from build123d import *

# Parameters (mm, degrees)
SKETCH1_W                                = 1524
SKETCH1_H                                = 152.4
BOSS_EXTRUDE1_DEPTH                      = 152.4
BOSS_EXTRUDE2_DEPTH                      = 152.4
FILLET1_R                                = 25.4
SKETCH9_W                                = 152.4
SKETCH9_H                                = 38.1
BOSS_EXTRUDE3_DEPTH                      = 101.6
SKETCH11_W                               = 152.4
SKETCH11_H                               = 38.1
BOSS_EXTRUDE4_DEPTH                      = 56.515
F_0000_CLEARANCE_HOLE1_D                 = 7.874
F_0000_CLEARANCE_HOLE1_DEPTH             = 12.7
F_0000_CLEARANCE_HOLE1_TIP               = 2.365588257
CBORE_FOR_3_4_HEX_HEAD_BOLT1_D           = 19.84248
CBORE_FOR_3_4_HEX_HEAD_BOLT1_CBORE_D     = 41.275
CBORE_FOR_3_4_HEX_HEAD_BOLT1_CBORE_DEPTH = 13.3096


with BuildPart() as part:
    # Sketch1 → Boss-Extrude1 (new body)
    with BuildSketch(Plane.XY):
        with Locations((762, 76.2)):
            Rectangle(SKETCH1_W, SKETCH1_H)
    extrude(amount=BOSS_EXTRUDE1_DEPTH)

    # Sketch8 → Boss-Extrude2 (add)
    with BuildSketch(Plane(origin=(0, 152.4, 0), x_dir=(1, 0, 0), z_dir=(0, 1, 0))):
        Polygon((0, -152.4), (-254, -355.6), (-286.356492461, -355.6), (-286.356492461, -152.4), (0, 0), align=None)
    boss_extrude2 = extrude(amount=-BOSS_EXTRUDE2_DEPTH)

    # Mirror1: Boss-Extrude2 across plane
    add(boss_extrude2.mirror(Plane(origin=(762, 0, 0), x_dir=(0, 0, 1), z_dir=(1, 0, 0))))

    # Fillet1
    # the kernel refuses this fillet: 25.4 mm, written as the material it takes off along each edge
    with BuildSketch(Plane(origin=(-342.412174328, 0, 182.23304427), x_dir=(0, 1, 0), z_dir=(0.882766643577138, 0, -0.4698117207856294))) as fillet1_piece_1:
        with BuildLine():
            CenterArc((FILLET1_R, FILLET1_R), FILLET1_R, 180, 90)
            Line((0, FILLET1_R), (0, 0))
            Line((0, 0), (FILLET1_R, 0))
        make_face()
    extrude(amount=451.385265964, mode=Mode.SUBTRACT)
    with BuildSketch(Plane(origin=(-286.356492461, 0, 419.1), x_dir=(0, 1, 0), z_dir=(0, 0, -1))) as fillet1_piece_2:
        with BuildLine():
            CenterArc((FILLET1_R, FILLET1_R), FILLET1_R, 180, 90)
            Line((0, FILLET1_R), (0, 0))
            Line((0, 0), (FILLET1_R, 0))
        make_face()
    extrude(amount=330.2, mode=Mode.SUBTRACT)
    with BuildSketch(Plane(origin=(49.5851694, 0, 112.73186448), x_dir=(0, 1, 0), z_dir=(-0.780868809443027, 0, 0.6246950475544286))) as fillet1_piece_3_section:
        with BuildLine():
            CenterArc((FILLET1_R, FILLET1_R), FILLET1_R, 180, 90)
            Line((0, FILLET1_R), (0, 0))
            Line((0, 0), (FILLET1_R, 0))
        make_face()
    fillet1_piece_3 = extrude(amount=452.278711262, mode=Mode.PRIVATE)
    fillet1_piece_3 = split(fillet1_piece_3, bisect_by=Plane(origin=(-158.082016781, 5.808462647, 152.4), z_dir=(0, 0, 1)), keep=Keep.TOP, mode=Mode.PRIVATE)
    add(fillet1_piece_3, mode=Mode.SUBTRACT)
    with BuildSketch(Plane(origin=(-63.5, 0, 152.4), x_dir=(0, 1, 0), z_dir=(1, 0, 0))) as fillet1_piece_4_section:
        with BuildLine():
            CenterArc((FILLET1_R, -FILLET1_R), FILLET1_R, 90, 90)
            Line((0, -FILLET1_R), (0, 0))
            Line((0, 0), (FILLET1_R, 0))
        make_face()
    fillet1_piece_4 = extrude(amount=1651, mode=Mode.PRIVATE)
    fillet1_piece_4 = split(fillet1_piece_4, bisect_by=Plane(origin=(467.415014496, 5.779770976, -221.532011596), z_dir=(0.6246950475544286, 0, 0.780868809443027)), keep=Keep.TOP, mode=Mode.PRIVATE)
    fillet1_piece_4 = split(fillet1_piece_4, bisect_by=Plane(origin=(1056.584985505, 5.779770976, -221.532011596), z_dir=(-0.6246950475544286, 0, 0.780868809443027)), keep=Keep.TOP, mode=Mode.PRIVATE)
    add(fillet1_piece_4, mode=Mode.SUBTRACT)
    with BuildSketch(Plane(origin=(1474.4148306, 0, 112.73186448), x_dir=(0, 1, 0), z_dir=(0.780868809443027, 0, 0.6246950475544286))) as fillet1_piece_5_section:
        with BuildLine():
            CenterArc((FILLET1_R, -FILLET1_R), FILLET1_R, 90, 90)
            Line((0, -FILLET1_R), (0, 0))
            Line((0, 0), (FILLET1_R, 0))
        make_face()
    fillet1_piece_5 = extrude(amount=452.278711262, mode=Mode.PRIVATE)
    fillet1_piece_5 = split(fillet1_piece_5, bisect_by=Plane(origin=(1682.082016781, 5.808462647, 152.4), z_dir=(0, 0, 1)), keep=Keep.TOP, mode=Mode.PRIVATE)
    add(fillet1_piece_5, mode=Mode.SUBTRACT)
    with BuildSketch(Plane(origin=(1810.356492461, 0, 419.1), x_dir=(0, 1, 0), z_dir=(0, 0, -1))) as fillet1_piece_6:
        with BuildLine():
            CenterArc((FILLET1_R, -FILLET1_R), FILLET1_R, 90, 90)
            Line((0, -FILLET1_R), (0, 0))
            Line((0, 0), (FILLET1_R, 0))
        make_face()
    extrude(amount=330.2, mode=Mode.SUBTRACT)
    with BuildSketch(Plane(origin=(1866.412174328, 0, 182.23304427), x_dir=(0, 1, 0), z_dir=(-0.882766643577138, 0, -0.4698117207856294))) as fillet1_piece_7:
        with BuildLine():
            CenterArc((FILLET1_R, -FILLET1_R), FILLET1_R, 90, 90)
            Line((0, -FILLET1_R), (0, 0))
            Line((0, 0), (FILLET1_R, 0))
        make_face()
    extrude(amount=451.385265964, mode=Mode.SUBTRACT)
    with BuildSketch(Plane(origin=(-63.5, 0, 0), x_dir=(0, 1, 0), z_dir=(1, 0, 0))) as fillet1_piece_8:
        with BuildLine():
            CenterArc((FILLET1_R, FILLET1_R), FILLET1_R, 180, 90)
            Line((0, FILLET1_R), (0, 0))
            Line((0, 0), (FILLET1_R, 0))
        make_face()
    extrude(amount=1651, mode=Mode.SUBTRACT)
    with BuildSketch(Plane(origin=(-63.5, 0, 152.4), x_dir=(0, 1, 0), z_dir=(1, 0, 0))) as fillet1_piece_9a_section:
        with BuildLine():
            CenterArc((FILLET1_R, -FILLET1_R), FILLET1_R, 90, 90)
            Line((0, -FILLET1_R), (0, 0))
            Line((0, 0), (FILLET1_R, 0))
        make_face()
    fillet1_piece_9a = extrude(amount=1651, mode=Mode.PRIVATE)
    fillet1_piece_9a = split(fillet1_piece_9a, bisect_by=Plane(origin=(-13.902468194, 5.43719391, 163.521974555), z_dir=(-0.6246950475544286, 0, -0.780868809443027)), keep=Keep.TOP, mode=Mode.PRIVATE)
    with BuildSketch(Plane(origin=(49.5851694, 0, 112.73186448), x_dir=(0, 1, 0), z_dir=(-0.780868809443027, 0, 0.6246950475544286))) as fillet1_piece_9b_section:
        with BuildLine():
            CenterArc((FILLET1_R, FILLET1_R), FILLET1_R, 180, 90)
            Line((0, FILLET1_R), (0, 0))
            Line((0, 0), (FILLET1_R, 0))
        make_face()
    fillet1_piece_9b = extrude(amount=452.278711262, mode=Mode.PRIVATE)
    fillet1_piece_9b = split(fillet1_piece_9b, bisect_by=Plane(origin=(17.80384621, 5.43719391, 152.4), z_dir=(0, 0, -1)), keep=Keep.TOP, mode=Mode.PRIVATE)
    fillet1_piece_9 = fillet1_piece_9a & fillet1_piece_9b
    add(fillet1_piece_9, mode=Mode.SUBTRACT)
    with BuildSketch(Plane(origin=(-63.5, 0, 152.4), x_dir=(0, 1, 0), z_dir=(1, 0, 0))) as fillet1_piece_10a_section:
        with BuildLine():
            CenterArc((FILLET1_R, -FILLET1_R), FILLET1_R, 90, 90)
            Line((0, -FILLET1_R), (0, 0))
            Line((0, 0), (FILLET1_R, 0))
        make_face()
    fillet1_piece_10a = extrude(amount=1651, mode=Mode.PRIVATE)
    fillet1_piece_10a = split(fillet1_piece_10a, bisect_by=Plane(origin=(1537.902468194, 5.43719391, 163.521974555), z_dir=(0.6246950475544286, 0, -0.780868809443027)), keep=Keep.TOP, mode=Mode.PRIVATE)
    with BuildSketch(Plane(origin=(1474.4148306, 0, 112.73186448), x_dir=(0, 1, 0), z_dir=(0.780868809443027, 0, 0.6246950475544286))) as fillet1_piece_10b_section:
        with BuildLine():
            CenterArc((FILLET1_R, -FILLET1_R), FILLET1_R, 90, 90)
            Line((0, -FILLET1_R), (0, 0))
            Line((0, 0), (FILLET1_R, 0))
        make_face()
    fillet1_piece_10b = extrude(amount=452.278711262, mode=Mode.PRIVATE)
    fillet1_piece_10b = split(fillet1_piece_10b, bisect_by=Plane(origin=(1506.19615379, 5.43719391, 152.4), z_dir=(0, 0, -1)), keep=Keep.TOP, mode=Mode.PRIVATE)
    fillet1_piece_10 = fillet1_piece_10a & fillet1_piece_10b
    add(fillet1_piece_10, mode=Mode.SUBTRACT)

    # Sketch9 → Boss-Extrude3 (add)
    with BuildSketch(Plane(origin=(0, 0, 0), x_dir=(-1, 0, 0), z_dir=(0, 0, -1))):
        with Locations((-457.2, 133.35)):
            Rectangle(SKETCH9_W, SKETCH9_H)
        with Locations((-1066.8, 133.35)):
            Rectangle(SKETCH9_W, SKETCH9_H)
    boss_extrude3 = extrude(amount=BOSS_EXTRUDE3_DEPTH)

    # Sketch11 → Boss-Extrude4 (add)
    with BuildSketch(Plane.ZY.offset(286.356492461)):
        with Locations((254, 133.35)):
            Rectangle(SKETCH11_W, SKETCH11_H)
    boss_extrude4 = extrude(amount=BOSS_EXTRUDE4_DEPTH)

    # Mirror3: Boss-Extrude4 across plane
    add(boss_extrude4.mirror(Plane(origin=(762, 0, 0), x_dir=(0, 0, 1), z_dir=(1, 0, 0))))

    # Mirror4: Boss-Extrude3 across plane
    add(boss_extrude3.mirror(Plane.XY.offset(76.2)))

    # #0000 Clearance Hole1
    with Locations(Plane(origin=(0, 0, 0), x_dir=(-1, 0, 0), z_dir=(0, -1, 0))):
        with Locations((222.856492461, -231.155200669), (19.656492461, -82.394199052), (-175.923507539, -76.2), (-371.503507539, -76.2), (-567.083507539, -76.2), (-762.028507539, -76.2), (-956.916492461, -76.2), (-1152.496492461, -76.2), (-1348.076492461, -76.2), (-1543.656492461, -76.2), (-1746.856492461, -231.155200669)):
            Hole(F_0000_CLEARANCE_HOLE1_D / 2, depth=F_0000_CLEARANCE_HOLE1_DEPTH)
            with Locations((0, 0, -(F_0000_CLEARANCE_HOLE1_DEPTH + F_0000_CLEARANCE_HOLE1_TIP / 2))):  # 118° drill point
                Cone(0, F_0000_CLEARANCE_HOLE1_D / 2, F_0000_CLEARANCE_HOLE1_TIP, mode=Mode.SUBTRACT)

    # CBORE for 3/4 Hex Head Bolt1 (through all)
    with Locations(Plane(origin=(0, 114.3, 0), x_dir=(-1, 0, 0), z_dir=(0, -1, 0))):
        with Locations((-457.2, 50.8), (-457.2, -203.2), (-1066.8, 50.8), (-1066.8, -203.2), (-1837.083507539, -254), (309.216492461, -254)):
            CounterBoreHole(CBORE_FOR_3_4_HEX_HEAD_BOLT1_D / 2, CBORE_FOR_3_4_HEX_HEAD_BOLT1_CBORE_D / 2, CBORE_FOR_3_4_HEX_HEAD_BOLT1_CBORE_DEPTH)


solid = part.part
Design review of the part built by this model. Coordinates are the model's own, in mm. A direction names the side the tool comes from. Round coordinates to 2 decimals unless told otherwise and drop trailing zeros. Loops run counter-clockwise (first coordinate to the right, second up) from the corner with the lowest first, then second, coordinate; pieces in that order, holes last. Notation, with made-up numbers: (42, 48.25) -> (48, 48.25) arc R29 ccw to (48, 76.25) -> close; hole circle Ø8 at (58, -11.75). An arc over 180 degrees is marked (long way). Use one line per item in the form item = value. Start each with the question number.
Q1. For pin 1 Ø4 at (y, z) = (55, 184.5) entering from -X; pin 2 Ø11.5 at (x, y) = (-313.5, 138) entering from -Z; pin 3 Ø6 at (x, z) = (1493.5, 148.5) entering from -Y; pin 4 Ø12.5 at (x, z) = (-222.86, 231.16) entering from -Y, all flat-tipped, find the tip position at first contact; note any pin that passes through.
Q2. Wall thickness on line 1 along Z through (x, y) = (1066.8, 120); line 2 along Z through (x, y) = (1375.5, 24.5); line 3 along Y through (x, z) = (1010, 12.5): over which ranges is each line inside the solid? List them lowest first. Write a range as [from, to].
Q3. Draft analysis for pull direction X (two halves, no side actions). For faces 1 (the face through (-145.183, 89.789, 77.267)), 2 (the face through (-304, 127.61, 263)), 3 (the face through (1838, 133, 177.8)), state which applies: +X half, -X half, draft (parallel to the pull), parting line (faces both ways), or undercut.
Q4. Machinability: for faces 4 (the face through (1857.7, 120.9, 253.1)), 5 (the face through (1143, 133, -50)), 6 (the face through (1851, 114.3, 236)), 7 (the face through (990.6, 133, 202)), 8 (the face through (990.6, 133, -50)), which of the approach directions +Z, -Z, +X, -X, +Y, -Y give a long, thin tool a straight path to every point of the face, cutting with its end or side? Answer none if there is none.
Q5. We need section A-A on x = 929.5. Give the boundary of the cut face in (y, z).
Calculated:
q1.pin_1 = -286.36
q1.pin_2 = 177.8
q1.pin_3 = 8
q1.pin_4 = 0
q2.line_1 = [-101.6, -71.44], [-30.16, 182.56], [223.84, 254]
q2.line_2 = [0.02, 152.38]
q2.line_3 = [3.52, 152.4]
q3.face_1 = -X half
q3.face_2 = undercut
q3.face_3 = draft
q4.face_4 = -Y
q4.face_5 = -Z, +X, +Y, -Y
q4.face_6 = +Z, -Z, +X, -Y
q4.face_7 = +Z, +Y, -Y
q4.face_8 = -Z, +Y, -Y
q5.outline = (0, 25.4) arc R25.4 ccw to (25.4, 0) -> (152.4, 0) -> (152.4, 152.4) -> (25.4, 152.4) arc R25.4 ccw to (0, 127) -> close
